Can you work these out from the model? Positions are in its coordinate system, mm. A direction names the side the tool comes from. Give positions to 0.01 mm unless a question says otherwise; leave off trailing zeros. Loops run counter-clockwise (first coordinate to the right, second up) from the corner with the lowest first, then second, coordinate; pieces in that order, holes last. Notation, with made-up numbers: (-39.5, -40) -> (17.5, -40) arc R36 cw to (17.5, -5) -> close; hole circle Ø11 at (73.25, 56.5). An arc over 180 degrees is marked (long way). Return JSON: item names as keys, results as strings. Group by question number.
Q1. Suppose I cut it at D-D, the plane z = 9.75. Count the separate pieces of the cut face and the enclosed holes in it, and give its area (3 significant figures).
Q2. Suppose I cut it at A-A, the plane x = 32.5. Please give me the cut outline in (y, z), and give its area (3 significant figures).
Q3. Which directions (+Z, -Z, +X, -X, +Y, -Y) give clear straight access to the entire face, cutting with the end or side of a thin tool? Please do faces 1 (the flat face through (-41.891, -9, 12)), 2 (the flat face through (34.55, -42.12, 12.32)), 3 (the flat face through (41.003, 19, 12)).
Q4. Thinking about a two-plate mould opening in Y: for faces 4 (the flat face through (31, 77.305, 12)), 5 (the flat face through (12.24, 99.73, 12.32)), 6 (the flat face through (-56, 25.609, 12)), which applies, pulls with the +Y half, pulls with the -Y half, needs draft (parallel to the pull), parting line crosses it, or undercut?
Q5. Suppose I cut it at B-B, the plane x = -23.5. Please give me the cut outline in (y, z), and give its area (3 significant figures).
Q6. I need wall thicknesses on line 1 along Y through (x, z) = (-13, 20.75); line 2 along Y through (x, z) = (-2.5, 16.25); line 3 along X through (y, z) = (-31.5, 5.5). Which ranges of each line are inside material? Lowest first, please. Write a range as [from, to].
Q7. Suppose I cut it at C-C, the plane y = -33.5. Please give me the cut outline in (x, z), and give its area (3 significant figures).
Q8. Will these pins go through, and if not, where does the flat tip stop? pin 1 (6 mm diameter, centred on x = -49.5, z = 7.5, fed in from +Y); pin 2 (7 mm diameter, centred on y = 20.5, z = 11.5, fed in from -X); pin 3 (12.5 mm diameter, centred on x = -49, z = 14.5, fed in from -Y).
```python
from build123d import *

# Parameters (mm, degrees)
F0_W     = 14.7602576762
F0_H     = 3.8799718022
F0_W_2   = 15.3383538127
F0_H_2   = 5.3616389632
F0_W_3   = 12.7302650362
F0_H_3   = 42.9276376963
F1_DEPTH = 25


with BuildPart() as f1:
    # F0 (on Top) → F1 (new body)
    with BuildSketch(Plane.XY):
        with BuildLine():
            Line((-41.8914481997, 25.6085544825), (-30.3453952074, 30.6414496154))
            Line((-30.3453952074, 30.6414496154), (-35.0931140335, 36.3630584026))
            ThreePointArc((-35.0931140335, 36.3630584026), (-36.1496783198, 40.5291275429), (-33.5824096079, 43.9760959986))
            Line((-33.5824096079, 43.9760959986), (-41.8914481997, 41.9146602538))
            Line((-41.8914481997, 41.9146602538), (-41.8914481997, 25.6085544825))
        make_face()
        Polygon((-30.2785868891, 25.6085544824), (-30.3453952074, 30.6414496154), (-41.8914481997, 25.6085544825), align=None)
        Polygon((-30.0270732639, 6.6611878574), (-30.2785868891, 25.6085544824), (-41.8914481997, 25.6085544825), (-41.8914481997, -45.4440824687), (-29.4572375715, -36.2664498389), align=None)
        Polygon((-69.4309175014, 25.6085544825), (-41.8914481997, 25.6085544825), (-41.8914481997, 41.9146602538), (-69.4309175014, 35.0822396576), align=None)
        Polygon((-29.4572375715, 87.4835588038), (-30.0270732639, 44.5559211075), (38.9467375503, 44.5559211075), align=None)
        with BuildLine():
            Line((-31.2453058591, 44.5559211075), (-30.0270732639, 44.5559211075))
            Line((-30.0270732639, 44.5559211075), (-29.4572375715, 87.4835588038))
            Line((-29.4572375715, 87.4835588038), (-41.8914481997, 96.6611914337))
            Line((-41.8914481997, 96.6611914337), (-41.8914481997, 41.9146602538))
            Line((-41.8914481997, 41.9146602538), (-33.5824096079, 43.9760959986))
            ThreePointArc((-33.5824096079, 43.9760959986), (-32.4492837544, 44.4088003794), (-31.2453058591, 44.5559211075))
        make_face()
        Polygon((-29.4572375715, -36.2664498389), (-41.8914481997, -45.4440824687), (28.2730255276, -45.4440824687), (28.2730255276, -36.2664498389), align=None)
        with BuildLine():
            Line((45.5025919776, 36.5155363053), (41.0032905638, 30.6414496154))
            Line((41.0032905638, 30.6414496154), (41.0032905638, 6.6611878574))
            Line((41.0032905638, 6.6611878574), (41.0032905638, -36.2664498389))
            Line((41.0032905638, -36.2664498389), (83.6994573474, 64.5043104887))
            Line((83.6994573474, 64.5043104887), (67.339964211, 117.6310479641))
            Line((67.339964211, 117.6310479641), (53.0811295514, 113.2402775379))
            Line((53.0811295514, 113.2402775379), (52.7791223524, 111.6383405707))
            Line((52.7791223524, 111.6383405707), (40.1323241217, 44.5559211075))
            Line((40.1323241217, 44.5559211075), (41.5332015641, 44.5559211075))
            ThreePointArc((41.5332015641, 44.5559211075), (46.0166112047, 41.7692981641), (45.5025919776, 36.5155363053))
        make_face()
        Polygon((-29.4572375715, 87.4835588038), (38.9467375503, 44.5559211075), (40.1323241217, 44.5559211075), (52.7791223524, 111.6383405707), align=None)
        with Locations((-7.3801288381, 83.009172231)):
            Rectangle(F0_W, F0_H, mode=Mode.SUBTRACT)
        with Locations((30.8985039592, 79.9858681858)):
            Rectangle(F0_W_2, F0_H_2, mode=Mode.SUBTRACT)
        with Locations((34.6381580457, -14.8026309907)):
            Rectangle(F0_W_3, F0_H_3)
        Polygon((28.2730255276, -36.2664498389), (28.2730255276, -45.4440824687), (28.2730255276, -47.8125028312), (41.0032905638, -36.2664498389), align=None)
    extrude(amount=F1_DEPTH)


solid = f1.part
```
Ans:
{
 "1": {"separate pieces": "1", "enclosed holes": "3", "area": "10,500 mm^2"},
 "2": {"outline": "(-43.98, 0) -> (6.66, 0) -> (6.66, 25) -> (-43.98, 25) -> close; (44.56, 0) -> (77.31, 0) -> (77.31, 25) -> (44.56, 25) -> close; (82.67, 0) -> (105.68, 0) -> (105.68, 25) -> (82.67, 25) -> close", "area": "2,660 mm^2"},
 "3": {"face 1": "+Z, -Z, -X, -Y", "face 2": "+Z, -Z, +X, -Y", "face 3": "+Z, -Z"},
 "4": {"face 4": "undercut", "face 5": "pulls with the +Y half", "face 6": "pulls with the -Y half"},
 "5": {"outline": "(-45.44, 0) -> (-36.27, 0) -> (-36.27, 25) -> (-45.44, 25) -> close; (44.56, 0) -> (89.23, 0) -> (89.23, 25) -> (44.56, 25) -> close", "area": "1,350 mm^2"},
 "6": {"line 1": "y = [-45.44, -36.27], [44.56, 81.07], [84.95, 92.32]", "line 2": "y = [-45.44, -36.27], [44.56, 81.07], [84.95, 95.4]", "line 3": "x = [-41.89, -29.52], [28.27, 43.02]"},
 "7": {"outline": "(-41.89, 0) -> (-29.49, 0) -> (-29.49, 25) -> (-41.89, 25) -> close; (28.27, 0) -> (42.18, 0) -> (42.18, 25) -> (28.27, 25) -> close", "area": "657 mm^2"},
 "8": {"pin 1": "stops at y = 40.77", "pin 2": "stops at x = -41.89", "pin 3": "stops at y = 25.61"}
}
